Study the drawing (mm; zero at the part's minimum x, y, z) and answer. Give positions to 0.01 mm unless a question says otherwise; leave off trailing zeros. Write each loop counter-clockwise with the first axis right and the second up, starting at its lowest first coordinate (ties: lowest second). Pieces come first, ordered by that corner, then holes. Notation, with made-up numbers: (-22.75, 46.25) - (-16.75, 46.25) arc R25 ccw to (-16.75, 69.25) - close; hole circle Ø5 at (-10.75, -26). An arc over 180 degrees is marked (long way). Write each question's results on one line, items separated by ' | '. Start each with the question number.
Q1. Section D-D (x = 44.5) is taken. Determine the outline of the cut face in (y, z) (3 decimals), plus the area to 3 significant figures.
Q2. A flat-ended cylindrical pin translates along its axis: pin 1 Ø4.5 at (x, z) = (37.211, 20.32) entering from -Y. Find the tip coordinate at first contact, or state that the pin passes through.
Q3. Section A-A (y = 0.6) is taken. State how many separate pieces and enclosed holes the cut face has, plus the area to 3 significant figures.
Q4. Find the intervals of material crossed by probe 1 along Z at (x, y) = (77.5, 0.3); probe 2 along Z at (x, y) = (86, 0.35), in increasing order.
Q5. Section B-B (x = 70.5) is taken. Determine the outline of the cut face in (y, z) (3 decimals).
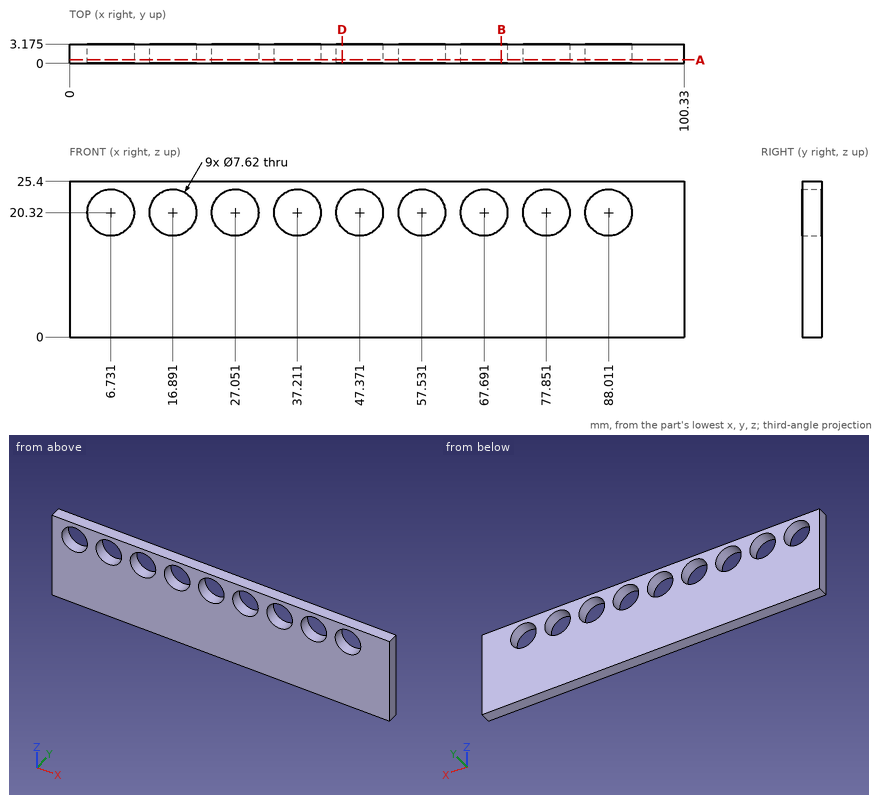
Answers below:
1) outline: (0, 0) - (3.175, 0) - (3.175, 17.815) - (0, 17.815) - close; (0, 22.825) - (3.175, 22.825) - (3.175, 25.4) - (0, 25.4) - close | area: 64.7 mm2
2) pin 1: passes through
3) separate pieces: 1 | enclosed holes: 9 | area: 2,140 mm2
4) probe 1: z = 0 to 16.53, 24.11 to 25.4 | probe 2: z = 0 to 17.08, 23.56 to 25.4
5) outline: (0, 0) - (3.175, 0) - (3.175, 17.746) - (0, 17.746) - close; (0, 22.894) - (3.175, 22.894) - (3.175, 25.4) - (0, 25.4) - close
